Geometry check sheet. Reference: the model listing, model coordinates, mm. A direction names the side the tool comes from. Round coordinates to 2 decimals unless told otherwise and drop trailing zeros. Order: outer loops, then holes, each group sorted by start corner. A loop starts at its lowest first (then second) coordinate and runs counter-clockwise, first axis right, second up. Notation, with made-up numbers: M -28.75,81 L -4.75,81 A24 cw -4.75,115 Z; hole C -19,32.5 d1. An arc over 180 degrees is marked long. Answer as a JSON object with one key per item and string values. Group by question number.
```python
from build123d import *

# Parameters (mm, degrees)
F0_W        = 88.978625834
F0_H        = 91.9070094824
F1_DEPTH    = 92.0228585601
F2_W        = 88.978625834
F2_H        = 91.9070094824
F3_DEPTH    = 64.5945444703
F4_T1_DEPTH = 353.1900010597
F5_W        = 26.5779765323
F5_H        = 57.0915937424
F6_DEPTH    = 3.2936800271
F8_W        = 21.8550208956
F8_H        = 52.9087015152
F9_DEPTH    = 3.0834991485
F10_R       = 12.2707310255
F11_DEPTH   = 1.7256960273
F12_DEPTH   = 0.6503686309


# Not quite as in the source:
# - a fillet or chamfer that OpenCascade refuses, or shapes differently, is made with other operations: its cross-section is extruded or revolved along the edge and cut away or added


with BuildPart() as f1:
    # F0 (on Top) → F1 (new body)
    with BuildSketch(Plane.XY):
        with Locations((-1.1190511286, 2.2303946316)):
            Rectangle(F0_W, F0_H)
    extrude(amount=F1_DEPTH)

    # F2 (on face) → F3 (join)
    with BuildSketch(Plane.XY.offset(92.0228585601)):
        with Locations((-1.1190511286, 2.2303946316)):
            Rectangle(F2_W, F2_H)
    extrude(amount=F3_DEPTH)

    # F4: chamfer of 50.8 on 2 edges, made by hand

    # F4_s2 → F4_t1 (cut)
    with BuildSketch(Plane.XZ.offset(-178.8253951615)):
        Polygon((-45.6083640456, 105.8174030304), (5.1916359544, 156.6174030304), (-45.6083640456, 156.6174030304), align=None)
        Polygon((43.3702617884, 105.8174030304), (-7.4297382116, 156.6174030304), (43.3702617884, 156.6174030304), align=None)
    extrude(amount=F4_T1_DEPTH, mode=Mode.SUBTRACT)

    # F5 (on face) → F6 (join)
    with BuildSketch(Plane(origin=(0, 48.1838993728, 0), x_dir=(-1, 0, 0), z_dir=(0, 1, 0))):
        with Locations((6.6281720065, 28.5457968712)):
            Rectangle(F5_W, F5_H)
    extrude(amount=F6_DEPTH)

    # F8 (on face) → F9 (join)
    with BuildSketch(Plane.XZ.offset(43.7231101096)):
        with Locations((-34.6808535978, 26.4543507576)):
            Rectangle(F8_W, F8_H)
    extrude(amount=F9_DEPTH)

    # F10 (on face) → F11 (join)
    with BuildSketch(Plane(origin=(0, 48.1838993728, 0), x_dir=(-1, 0, 0), z_dir=(0, 1, 0))):
        with Locations((0, 125.5997568369)):
            Circle(F10_R)
    extrude(amount=F11_DEPTH)

    # F12 (add): a face of the model
    f12_faces = [f1.faces().sort_by_distance(p)[0] for p in [
        (0, 49.9095954001, 125.5997568369),
    ]]
    extrude(f12_faces, amount=F12_DEPTH)


solid = f1.part
```
1) Sectioned sample at D-D (x = 22.5). Record the boundary of the cut face in (y, z).
2) Sectioned sample at A-A (z = 40). Record the boundary of the cut face in (x, y), then the cut area to 3 significant figures.
3) Go/stop test with flat-tipped pins: P1, Ø0.9, axis at y = -45.5, z = 26.5, coming from the +X side; P2, Ø1, axis at x = -27, y = 2.5, coming from the +Z side; P3, Ø6, axis at x = 5.5, z = 20.5, coming from the -Y side. Record where each tip stops, or that it passes through.
4) Set-up check for faces 1 (the flat face through (-35, -45, 52.909)), 2 (the flat face through (-19.917, 50, 28)), 3 (the flat face through (-6, 50, 57.092)), 4 (the flat face through (0, 50.56, 126)), 5 (the flat face through (6.661, 50, 28)): record each of +Z, -Z, +X, -X, +Y, -Y from which the full face is reachable in a straight line by a thin tool's end or side.
5) Release check for a two-part mould opening along Z. For faces 6 (the flat face through (-45.608, 1, 52)), 7 (the flat face through (-1.7, 48.184, 57.4)), 8 (the flat face through (21.44, 2.87, 127.75)) record: +Z half, -Z half, draft (parallel to the pull), parting line (faces both ways), or undercut.
6) Thickness scan on line 1 along Y through (x, z) = (28, 30); line 2 along Y through (x, z) = (-14, 49); line 3 along Z through (x, y) = (30.5, -11.5). Record the ranges inside material, lowest first. Write a range as [from, to].
7) Sectioned sample at C-C (x = -31.5). Record the boundary of the cut face in (y, z).
8) Sectioned sample at B-B (y = 10.5). Record the boundary of the cut face in (x, z).
Final values:
{
 "1": {"outline": "M -43.72,0 L 48.18,0 L 48.18,126.69 L -43.72,126.69 Z"},
 "2": {"outline": "M -45.61,-46.81 L -23.75,-46.81 L -23.75,-43.72 L 43.37,-43.72 L 43.37,48.18 L 6.66,48.18 L 6.66,51.48 L -19.92,51.48 L -19.92,48.18 L -45.61,48.18 Z", "area": "8,330 mm^2"},
 "3": {"P1": "stops at x = -23.75", "P2": "stops at z = 124.93", "P3": "stops at y = -43.72"},
 "4": {"face 1": "+Z, +X, -X, -Y", "face 2": "+Z, -Z, -X, +Y", "face 3": "+X, -X, +Y", "face 4": "+Z, +X, -X, +Y", "face 5": "-Z, +X, +Y"},
 "5": {"face 6": "draft", "face 7": "undercut", "face 8": "+Z half"},
 "6": {"line 1": "y = [-43.72, 48.18]", "line 2": "y = [-43.72, 51.48]", "line 3": "z = [0, 118.69]"},
 "7": {"outline": "M -46.81,0 L 48.18,0 L 48.18,119.93 L -43.72,119.93 L -43.72,52.91 L -46.81,52.91 Z"},
 "8": {"outline": "M -45.61,0 L 43.37,0 L 43.37,105.82 L -1.12,150.31 L -45.61,105.82 Z"}
}
